Verification items for the finished model (mm, model axes). A direction names the side the tool comes from. Round coordinates to 2 decimals unless told otherwise and drop trailing zeros. Order: outer loops, then holes, each group sorted by start corner. A loop starts at its lowest first (then second) coordinate and runs counter-clockwise, first axis right, second up. Notation, with made-up numbers: (-25, 65.5) -> (23, 65.5) arc R28 cw to (23, 90.5) -> close; hole circle Ø10 at (43.25, -33.5). An arc over 180 degrees is marked (long way). Return JSON: item names as keys, results as strings. Group by question number.
1) Section check B-B on x = -32.5. Enter the section's corners in (y, z), plus the area to 3 significant figures.
2) Section check C-C on x = -7.5. Enter the section's corners in (y, z).
3) Scan lines: L1, parallel to X at y = 0.75, z = 7.5; L2, parallel to X at y = 2, z = 22.5; L3, parallel to Z at x = -17.5, y = 1.8. Record each from-to range of solid material in increasing order.
4) Draft check along X on faces 3 (the cylindrical face through (-37.344, 1.521, 14.947)), 4 (the cylindrical face through (-33.38, 1.48, 6.35)), 5 (the flat face through (-15, 3, 14)), 6 (the flat face through (-23.351, 1.521, 23.492)). Enter one of: pulls with the +X half, pulls with the -X half, needs draft (parallel to the pull), parting line crosses it, or undercut.
5) Section check A-A on z = 32.5. Enter the section's corners in (x, y).
6) Section check D-D on z = 22.5. Enter the section's corners in (x, y), plus the area to 3 significant figures.
7) Depth check by flat-ended pin: pin 1 (2.5 mm diameter, centred on x = -22.5, z = 7.5, fed in from +Y); pin 2 (1 mm diameter, centred on y = 1, z = 26, fed in from -X); pin 3 (4.5 mm diameter, centred on x = -7.5, z = 32.5, fed in from -Y). Enter the tip coordinate at first touch or a pass-through.
8) Tool access check on faces 1 (the flat face through (-26.4, 1.5, 26.1)), 2 (the flat face through (-15, 1, 22)). Record the directions out of +Z, -Z, +X, -X, +Y, -Y that give a thin tool (end or side, any length) a straight path to the whole face; none if there is none.
```python
from build123d import *

# Parameters (mm, degrees)
SKETCH_1_R      = 1.45
EXTRUDE_1_DEPTH = 3
EXTRUDE_2_DEPTH = 3
FILLET_1_R      = 2


with BuildPart() as part:
    # 草图1 → 凸台-拉伸1 (new body)
    with BuildSketch(Plane(origin=(0, 0, 0), x_dir=(1, 0, 0), z_dir=(0, 1, 0))):
        Polygon((0, 0), (-37.5, 0), (-37.5, -15), (-15, -15), (-15, -37.5), (0, -37.5), align=None)
        with Locations(Location((-7.5, -7.5, 0), (0, 0, 270))):
            Circle(SKETCH_1_R, mode=Mode.SUBTRACT)
        with Locations(Location((-22.5, -7.5, 0), (0, 0, 270))):
            Circle(SKETCH_1_R, mode=Mode.SUBTRACT)
        with Locations(Location((-32.5, -7.5, 0), (0, 0, 270))):
            Circle(SKETCH_1_R, mode=Mode.SUBTRACT)
        with Locations(Location((-7.5, -22.5, 0), (0, 0, 270))):
            Circle(SKETCH_1_R, mode=Mode.SUBTRACT)
        with Locations(Location((-7.5, -32.5, 0), (0, 0, 270))):
            Circle(SKETCH_1_R, mode=Mode.SUBTRACT)
    extrude(amount=EXTRUDE_1_DEPTH)

    # 草图2 → 凸台-拉伸2 (add)
    with BuildSketch(Plane(origin=(0, 3, 0), x_dir=(1, 0, 0), z_dir=(0, 1, 0))):
        Polygon((-37.5, -15), (-15, -37.5), (-15, -31.843145751), (-31.843145751, -15), align=None)
    extrude(amount=-EXTRUDE_2_DEPTH)

    # 圆角1
    fillet_1_edges = [part.edges().sort_by_distance(p)[0] for p in [
        (0, 1.5, 37.5),
        (-15, 1.5, 37.5),
        (-15, 1.5, 15),
        (-37.5, 1.5, 15),
        (-37.5, 1.5, 0),
        (0, 1.5, 0),
        (-31.843145751, 1.5, 15),
        (-15, 1.5, 31.843145751),
    ]]
    fillet(fillet_1_edges, radius=FILLET_1_R)


solid = part.part
```
Check result:
{
 "1": {"outline": "(0, 0) -> (3, 0) -> (3, 6.05) -> (0, 6.05) -> close; (0, 8.95) -> (3, 8.95) -> (3, 20) -> (0, 20) -> close", "area": "51.3 mm^2"},
 "2": {"outline": "(0, 0) -> (3, 0) -> (3, 6.05) -> (0, 6.05) -> close; (0, 8.95) -> (3, 8.95) -> (3, 21.05) -> (0, 21.05) -> close; (0, 23.95) -> (3, 23.95) -> (3, 31.05) -> (0, 31.05) -> close; (0, 33.95) -> (3, 33.95) -> (3, 37.5) -> (0, 37.5) -> close"},
 "3": {"L1": "-37.5 to -33.95, -31.05 to -23.95, -21.05 to -8.95, -6.05 to 0", "L2": "-30 to -24.34, -15 to -8.95, -6.05 to 0", "L3": "0 to 15, 28.95 to 35"},
 "4": {"face 3": "pulls with the -X half", "face 4": "undercut", "face 5": "needs draft", "face 6": "undercut"},
 "5": {"outline": "(-20, 0) -> (-8.95, 0) -> (-8.95, 3) -> (-20, 3) -> close; (-6.05, 0) -> (0, 0) -> (0, 3) -> (-6.05, 3) -> close"},
 "6": {"outline": "(-30, 0) -> (-24.34, 0) -> (-24.34, 3) -> (-30, 3) -> close; (-15, 0) -> (-8.95, 0) -> (-8.95, 3) -> (-15, 3) -> close; (-6.05, 0) -> (0, 0) -> (0, 3) -> (-6.05, 3) -> close", "area": "53.3 mm^2"},
 "7": {"pin 1": "through", "pin 2": "x = -27", "pin 3": "y = 0"},
 "8": {"face 1": "+Z, -X, +Y, -Y", "face 2": "+Y, -Y"}
}
